The model under review builds one solid part; all positions refer to its coordinate system, in mm. Face numbers are marked on the shaded views. A direction names the side the tool comes from. Give positions to 0.01 mm unless a question says otherwise; leave off trailing zeros. Loops run counter-clockwise (first coordinate to the right, second up) from the corner with the lowest first, then second, coordinate; pieces in that order, holes last. Notation, with made-up numbers: M 82,85 L 130,85 A8 cw 130,100 Z; hole C 64,-21 d6. An arc over 180 degrees is marked long. Return JSON: item names as keys, results as strings.
```python
from build123d import *

# Parameters (mm, degrees)
F0_W     = 15.706341
F0_H     = 20
F1_DEPTH = 60
F2_DEPTH = 40
F3_DEPTH = 20


with BuildPart() as f1:
    # F0 (on Front) → F1 (new body)
    with BuildSketch(Plane.XZ):
        Polygon((0, 20), (0, 0), (100, 0), (100, 10), (15.706341, 10), (15.706341, 20), align=None)
        with Locations((7.853171, 30)):
            Rectangle(F0_W, F0_H)
        Polygon((15.706341, 40), (15.706341, 20), (15.706341, 10), (100, 10), (100, 30), (70, 30), (70, 40), align=None)
    extrude(amount=-F1_DEPTH)

    # F0 (on Front) → F2 (cut)
    with BuildSketch(Plane.XZ):
        Polygon((15.706341, 40), (15.706341, 20), (15.706341, 10), (100, 10), (100, 30), (70, 30), (70, 40), align=None)
    extrude(amount=-F2_DEPTH, mode=Mode.SUBTRACT)

    # F0 (on Front) → F3 (cut)
    with BuildSketch(Plane.XZ):
        with Locations((7.853171, 30)):
            Rectangle(F0_W, F0_H)
    extrude(amount=-F3_DEPTH, mode=Mode.SUBTRACT)


solid = f1.part
```
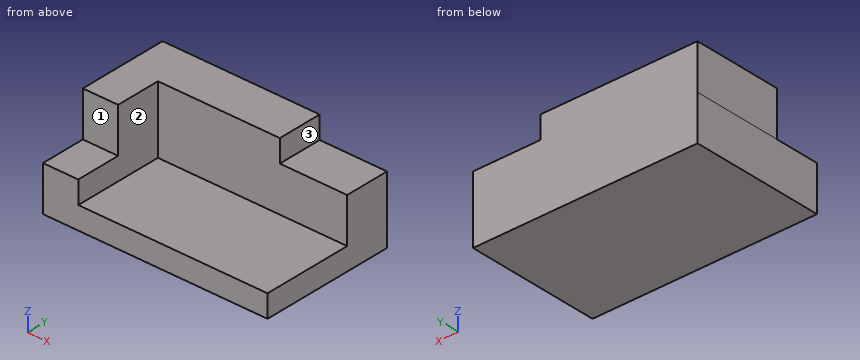
1) Consider section C-C on x = 12.5. Write out the cut boundary in (y, z), then the cut area to 3 significant figures.
From the geometry:
{"outline": "M 0,0 L 60,0 L 60,40 L 20,40 L 20,20 L 0,20 Z", "area": "2,000 mm²"}
2) Consider section A-A on y = 54.5. Write out the cut boundary in (x, z).
From the geometry:
{"outline": "M 0,0 L 100,0 L 100,30 L 70,30 L 70,40 L 0,40 Z"}
3) Wall thickness on L1, parallel to Y at x = 76, z = 26; L2, parallel to Z at x = 48.5, y = 8; L3, parallel to Z at x = 10, y = 12.5: over which ranges is each line inside the solid? List them lowest first. Write a range as from..to.
From the geometry:
{"L1": "40..60", "L2": "0..10", "L3": "0..20"}
4) Consider section D-D on y = 31. Write out the cut boundary in (x, z).
From the geometry:
{"outline": "M 0,0 L 100,0 L 100,10 L 15.71,10 L 15.71,40 L 0,40 Z"}
5) Tool access review of the marked faces 1, 2 and 3: name each direction out of +Z, -Z, +X, -X, +Y, -Y from which nothing blocks a thin tool from reaching the whole face with its end or side.
From the geometry:
{"face 1": "+Z, +X, -X, -Y", "face 2": "+Z, +X, -Y", "face 3": "+Z, +X, +Y, -Y"}
6) Insertion check: pin 1 (16 mm diameter, centred on x = 84, y = 50.5, fed in from +Z); pin 2 (3 mm diameter, centred on x = 36.5, y = 27, fed in from +Z); pin 3 (15 mm diameter, centred on y = 17.5, z = 26.5, fed in from +X); pin 4 (8 mm diameter, centred on y = 15.5, z = 35.5, fed in from +X). Each pin has a flat end and moves straight along its axis. Give the tip position at first contact, or say it passes through.
From the geometry:
{"pin 1": "z = 30", "pin 2": "z = 10", "pin 3": "x = 15.71", "pin 4": "through"}
7) Consider section B-B on z = 15. Write out the cut boundary in (x, y).
From the geometry:
{"outline": "M 0,0 L 15.71,0 L 15.71,40 L 100,40 L 100,60 L 0,60 Z"}
